Build history of the part. All positions in model axes, mm. A direction names the side the tool comes from. Give positions to 0.01 mm unless a question says otherwise; leave off trailing zeros. Order: outer loops, then holes, each group sorted by start corner. A loop starts at its lowest first (then second) coordinate and runs counter-clockwise, first axis right, second up. Notation, with made-up numbers: (6, 23) - (26, 23) arc R13 cw to (26, 41) - close; hole circle Ø4 at (-18.5, 87.5). An arc over 180 degrees is marked (long way). Use a Markdown table: item, result.
Autodesk Inventor part; units mm, degrees
ref_plane "YZ Plane" through (0, 0, 0) normal (1, 0, 0) x (0, 1, 0)
ref_plane "XZ Plane" through (0, 0, 0) normal (0, 1, 0) x (-1, 0, 0)
ref_plane "XY Plane" through (0, 0, 0) normal (0, 0, 1) x (1, 0, 0)
sketch "Esboço1" plane through (0, 0, 0) normal (0, 1, 0) x (-1, 0, 0)
  line L0 (0, 0) -> (32, 0)
  line L1 (32, 0) -> (32, -30)
  line L2 (32, -30) -> (0, -30)
  line L3 (0, -30) -> (0, 0)
  dimension "d0" = 32
  dimension "d1" = 30
extrude "Extrusion1" add sketch "Esboço1" along normal blind 5
sketch "Sketch4" plane through (0, 5, 0) normal (0, 1, 0) x (1, 0, 0)
  line L0 (-32, 30) -> (-28, 30)
  line L1 (-28, 30) -> (-28, 0)
  line L2 (-28, 0) -> (-32, 0)
  line L3 (-32, 0) -> (-32, 30)
  line L4 (-4, 30) -> (0, 30)
  line L5 (0, 30) -> (0, 0)
  line L6 (0, 0) -> (-4, 0)
  line L7 (-4, 0) -> (-4, 30)
  dimension "d59" = 24
extrude "Extrusion2" add sketch "Sketch4" along normal blind 26
sketch "Sketch5" plane through (0, 0, 0) normal (1, 0, 0) x (0, 0, -1)
  line L0 (0, 0) -> (0, 31)
  line L1 (30, 0) -> (30, 31)
  line L2 (0, 31) -> (30, 31)
  point P0 (7.5, 18)
  point P1 (22.5, 18)
  dimension "d30" = 7.5
  dimension "d31" = 7.5
  dimension "d32" = 13
  dimension "d33" = 13
hole "Hole2" at (0, 18, -7.5) at (0, 18, -22.5) direction (-1, 0, 0) diameter 5 end through all
sketch "Esboço6" plane through (0, 5, 0) normal (0, 1, 0) x (1, 0, 0)
  line L0 (-4, 30) -> (-28, 30)
  line L1 (-28, 0) -> (-28, 30)
  line L2 (-32, 30) -> (-32, 0)
  line L3 (-4, 30) -> (-4, 0)
  point P0 (0, 0)
  point P1 (-16, 22.5)
  point P2 (-16, 7.5)
  dimension "d43" = 15
  dimension "d45" = 24
  dimension "d48" = 30
  dimension "d57" = 12
  dimension "d58" = 7.5
hole "Furo3" at (-16, 5, -22.5) at (-16, 5, -7.5) direction (0, -1, 0) diameter 4 depth 5
equation "\"d39\" = Espessura"
equation "\"d55\" = Espessura"
equation "\"Raio_vergadura\" = Espessura"
equation "\"Largura_alívio_de_vergadura\" = Espessura"
equation "\"Profundidade_alívio_de_vergadura\" = 0.5 * Espessura"
equation "\"Raiodetransição\" = Raio_vergadura"
equation "\"Tamanho_de_raio_de_Jacobi\" = Raio_vergadura"
equation "\"TamanhoFolga\" = Espessura"
properties part number "Suporte da célula de carga" material "Aço galvanizado"
1) Slice it at C-C (x = -16). Write the cut outline in (y, z), and give its area (3 significant figures).
Computed:
| item | result |
|---|---|
| outline | (0, -30) - (5, -30) - (5, -24.5) - (0, -24.5) - close; (0, -20.5) - (5, -20.5) - (5, -9.5) - (0, -9.5) - close; (0, -5.5) - (5, -5.5) - (5, 0) - (0, 0) - close |
| area | 110 mm² |
2) Slice it at B-B (y = 18). Write the cut outline in (x, z).
Computed:
| item | result |
|---|---|
| outline | (-32, -30) - (-28, -30) - (-28, -25) - (-32, -25) - close; (-32, -20) - (-28, -20) - (-28, -10) - (-32, -10) - close; (-32, -5) - (-28, -5) - (-28, 0) - (-32, 0) - close; (-4, -30) - (0, -30) - (0, -25) - (-4, -25) - close; (-4, -20) - (0, -20) - (0, -10) - (-4, -10) - close; (-4, -5) - (0, -5) - (0, 0) - (-4, 0) - close |
3) Wall check: line 1 (Z direction, x = -1.9, y = 18); line 2 (Z direction, x = -16, y = 1.4); line 3 (X direction, y = 19, z = -2.25). Give the ranges that are in metal, low to high. Write a range as from..to.
Computed:
| item | result |
|---|---|
| line 1 | z = -30..-25, -20..-10, -5..0 |
| line 2 | z = -30..-24.5, -20.5..-9.5, -5.5..0 |
| line 3 | x = -32..-28, -4..0 |
4) Slice it at A-A (z = -7.5). Write the cut outline in (x, y).
Computed:
| item | result |
|---|---|
| outline | (-32, 0) - (-18, 0) - (-18, 5) - (-28, 5) - (-28, 15.5) - (-32, 15.5) - close; (-32, 20.5) - (-28, 20.5) - (-28, 31) - (-32, 31) - close; (-14, 0) - (0, 0) - (0, 15.5) - (-4, 15.5) - (-4, 5) - (-14, 5) - close; (-4, 20.5) - (0, 20.5) - (0, 31) - (-4, 31) - close |
5) Two-plate mould, pull along X, no slides. Class faces 3 (the flat face through (0, 15, -15)), 4 (the cylindrical face through (-2.028, 17.249, -9.885)), 5 (the flat face through (-4, 18, -15)), 6 (the flat face through (-28, 18, -15)): +X half, -X half, draft (parallel to the pull), parting line (faces both ways), or undercut.
Computed:
| item | result |
|---|---|
| face 3 | +X half |
| face 4 | draft |
| face 5 | undercut |
| face 6 | undercut |
6) Pin check, flat tip, straight feed: P1, Ø7, axis at x = -19.5, z = -21, coming from the +Y side. Stop position of the tip, or through.
Computed:
| item | result |
|---|---|
| P1 | stops at y = 5 |
7) Tool access for faces 1 (the flat face through (-16, 0, -15)), 2 (the flat face through (-16, 5, -15)): list every direction of +Z, -Z, +X, -X, +Y, -Y with a clear straight run to the whole face (end or side of a thin tool).
Computed:
| item | result |
|---|---|
| face 1 | +Z, -Z, +X, -X, -Y |
| face 2 | +Z, -Z, +Y |
8) Slice it at D-D (z = -17.5). Write the cut outline in (x, y).
Computed:
| item | result |
|---|---|
| outline | (-32, 0) - (0, 0) - (0, 31) - (-4, 31) - (-4, 5) - (-28, 5) - (-28, 31) - (-32, 31) - close |
